```python
from build123d import *

# Parameters (mm, degrees)
F0_W     = 203.2
F0_H     = 203.2
F0_R     = 3.175
F0_W_2   = 165.100006
F0_H_2   = 165.100005
F1_DEPTH = 19.05


with BuildPart() as f1:
    # F0 (on Top) → F1 (new body)
    with BuildSketch(Plane.XY):
        with Locations((-37.103736, 42.032712)):
            Rectangle(F0_W, F0_H)
        with Locations((-88.174261, -48.707619)):
            Circle(F0_R, mode=Mode.SUBTRACT)
        with Locations((-37.103736, 42.032713)):
            Rectangle(F0_W_2, F0_H_2, mode=Mode.SUBTRACT)
        with Locations((0, 137.821719)):
            Circle(F0_R, mode=Mode.SUBTRACT)
    extrude(amount=F1_DEPTH)


solid = f1.part
```
For this review, take the finished solid that the model builds, in its own axes (mm). A direction names the side the tool comes from. Round coordinates to 2 decimals unless told otherwise and drop trailing zeros. Write each loop counter-clockwise with the first axis right and the second up, starting at its lowest first coordinate (ties: lowest second). Pieces come first, ordered by that corner, then holes. Notation, with made-up numbers: M 71,-18 L 91,-18 A22 cw 91,-11 Z; hole C -6.75,50 d6. An arc over 180 degrees is marked long. One line per item, written item: value. Start each with the question number.
(1) We need section D-D (z = 11.5). Give the boundary of the cut face in (x, y) (3 decimals), and give its area (3 significant figures).
(2) Machinability: for faces 5 (the flat face through (-38, -40.517, 9)), 6 (the flat face through (-39, 143.633, 9)), which of the approach directions +Z, -Z, +X, -X, +Y, -Y give a long, thin tool a straight path to every point of the face, cutting with its end or side? Answer none if there is none.
(3) Wall thickness on line 1 (Y direction, x = 0, z = 6.5); line 2 (X direction, y = 14, z = 7.5); line 3 (Y direction, x = -5, z = 1.75): over which ranges is each line inside the solid? List them lowest first.
(4) Insertion check: pin 1 (5.5 mm diameter, centred on x = -88.17, y = -48.71, fed in from +Z). The pin has a flat end and moves straight along its axis. Give the tip position at first contact, or say it passes through.
(5) The part is to be moulded in two halves that separate along X. For faces 1 (the cylindrical face through (-0.41, 140.97, 9.39)), 2 (the flat face through (64.496, 41, 9)), 3 (the flat face through (-119.654, 41, 9)), 4 (the flat face through (52, 43, 19.05)), say which applies: released by +X, released by -X, zero draft, split by the parting line, or undercut.
(6) We need section B-B (y = 73). Give the boundary of the cut face in (x, z), and give its area (3 significant figures).
(7) We need section C-C (x = 0). Give the boundary of the cut face in (y, z).
(8) We need section A-A (x = 21). Give the boundary of the cut face in (y, z).
Result:
1. outline: M -138.704,-59.567 L 64.496,-59.567 L 64.496,143.633 L -138.704,143.633 Z; hole M -119.654,-40.517 L 45.446,-40.517 L 45.446,124.583 L -119.654,124.583 Z; hole C -88.174,-48.708 d6.35; hole C 0,137.822 d6.35
1. area: 14,000 mm²
2. face 5: +Z, -Z
2. face 6: +Z, -Z, +X, -X, +Y
3. line 1: -59.57 to -40.52, 124.58 to 134.65, 141 to 143.63
3. line 2: -138.7 to -119.65, 45.45 to 64.5
3. line 3: -59.57 to -40.52, 124.58 to 143.63
4. pin 1: through
5. face 1: undercut
5. face 2: released by +X
5. face 3: undercut
5. face 4: zero draft
6. outline: M -138.7,0 L -119.65,0 L -119.65,19.05 L -138.7,19.05 Z; M 45.45,0 L 64.5,0 L 64.5,19.05 L 45.45,19.05 Z
6. area: 726 mm²
7. outline: M -59.57,0 L -40.52,0 L -40.52,19.05 L -59.57,19.05 Z; M 124.58,0 L 134.65,0 L 134.65,19.05 L 124.58,19.05 Z; M 141,0 L 143.63,0 L 143.63,19.05 L 141,19.05 Z
8. outline: M -59.57,0 L -40.52,0 L -40.52,19.05 L -59.57,19.05 Z; M 124.58,0 L 143.63,0 L 143.63,19.05 L 124.58,19.05 Z
